Job drawing, mm, ordinate dimensions from the low corner. One solid piece. A direction names the side the tool comes from. Coordinates: 2 decimals unless noted, no trailing zeros. Order: outer loops, then holes, each group sorted by start corner. A loop starts at its lowest first (then second) coordinate and runs counter-clockwise, first axis right, second up. Notation, with made-up numbers: (55, 26) - (100, 26) arc R14 cw to (100, 35) - close; hole circle Ø8 at (48, 33.25). An arc over 180 degrees is marked (long way). Write each question's results on one line, items separated by ' | '. Start each with the question number.
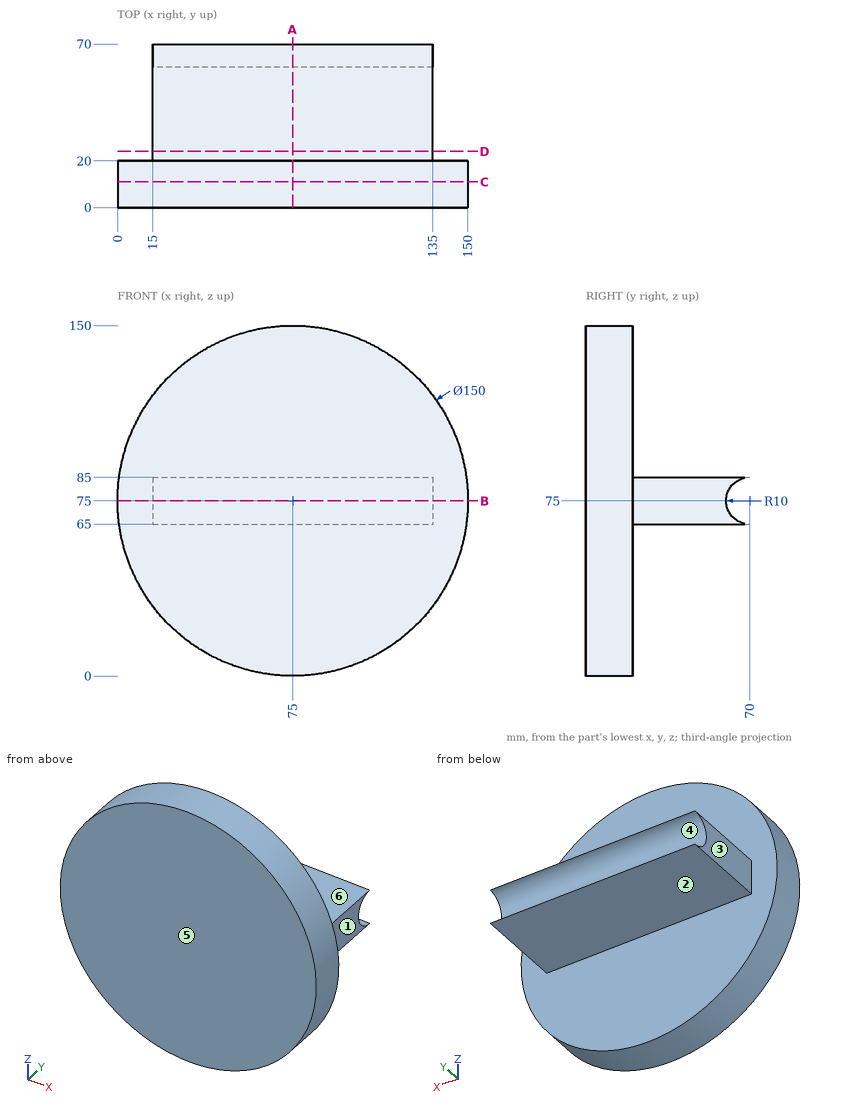
Item 1: Slice it at C-C (y = 11). Write the cut outline in (x, z), then the cut area to 3 significant figures.
Item 2: Probe probe 1 along X at (y, z) = (50.5, 68); probe 2 along Z at (x, y) = (18.5, 42); probe 3 along Y at (x, z) = (103.5, 39). List the from-to ranges inside material, lowest first.
Item 3: Pull direction Z, two halves, no side cores. Call the marked faces 4, 5 and 6: released by +Z, released by -Z, zero draft, split by the parting line, or undercut.
Item 4: Which spindle directions (+Z, -Z, +X, -X, +Y, -Y) get a long thin tool onto all of the face, cutting with end or side? Do the marked faces 1, 2 and 3. Say none if no direction does.
Item 5: Flat gauge pins, fed straight in: P1, Ø3, axis at x = 98, y = 15, coming from the -Z side; P2, Ø4, axis at x = 70.5, z = 72.5, coming from the -Y side; P3, Ø1, axis at x = 134, y = 48, coming from the +Z side; P4, Ø10, axis at y = 38, z = 75.5, coming from the +X side. Where does each tip first touch, or does it go through?
Item 6: Slice it at D-D (y = 24). Write the cut outline in (x, z).
Item 7: Slice it at B-B (z = 75). Write the cut outline in (x, y), then the cut area to 3 significant figures.
Item 8: Slice it at A-A (x = 75). Write the cut outline in (y, z).
Resolved:
1) outline: circle Ø150 at (75, 75) | area: 17,700 mm^2
2) probe 1: 15 to 135 | probe 2: 65 to 85 | probe 3: 0 to 20
3) face 4: undercut | face 5: zero draft | face 6: released by +Z
4) face 1: +Z, -Z, +X, +Y | face 2: -Z, +X, -X, +Y | face 3: +Z, -Z, -X, +Y
5) P1: z = 3.15 | P2: y = 0 | P3: z = 85 | P4: x = 135
6) outline: (15, 65) - (135, 65) - (135, 85) - (15, 85) - close
7) outline: (0, 0) - (150, 0) - (150, 20) - (135, 20) - (135, 60) - (15, 60) - (15, 20) - (0, 20) - close | area: 7,800 mm^2
8) outline: (0, 0) - (20, 0) - (20, 65) - (70, 65) arc R10 cw to (70, 85) - (20, 85) - (20, 150) - (0, 150) - close
